Part model, mm, in its own coordinate system. A direction names the side the tool comes from. Give positions to 0.01 mm unless a question says otherwise; leave off trailing zeros. Write each loop counter-clockwise with the first axis right and the second up, starting at its lowest first coordinate (ties: lowest second). Pieces come first, ordered by that corner, then holes.
Autodesk Inventor part; units mm, degrees
ref_plane "YZ Plane" through (0, 0, 0) normal (1, 0, 0) x (0, 1, 0)
ref_plane "XZ Plane" through (0, 0, 0) normal (0, 1, 0) x (-1, 0, 0)
ref_plane "XY Plane" through (0, 0, 0) normal (0, 0, 1) x (1, 0, 0)
sketch "Esboço1" plane through (0, 0, 0) normal (0, 0, 1) x (1, 0, 0)
  circle A0 centre (0, 0) radius 10
  dimension "d0" = 20
extrude "Extrusão1" add sketch "Esboço1" along normal mid plane 300
sketch "Esboço2" plane through (0, 0, 150) normal (0, 0, 1) x (1, 0, 0)
  circle A0 centre (0, 0) radius 8
  dimension "d3" = 16
extrude "Extrusão2" add sketch "Esboço2" along normal blind 40
fillet "Arredondamento1" radius 2 1 edges at (-8, 0, 190)
mirror "Espelhamento1" about plane through (0, 0, 0) normal (0, 0, 1) of "Extrusão2", "Arredondamento1"
properties part number "Haste da Morsa"
1) Drill centre lines: L1, parallel to Z at x = 1, y = 9; L2, parallel to Y at x = -0.75, z = 60; L3, parallel to X at y = -0.75, z = 167.5. Where is each one in solid material? Low to high.
Check result:
L1: z = -150 to 150
L2: y = -9.97 to 9.97
L3: x = -7.96 to 7.96
2) 3-axis set-ups, long thin cutter, end or side, ignore diameter. For faces 1 (the cylindrical face through (-1.73, -7.81, -168.73)), 2 (the cylindrical face through (-1.73, 7.81, 168.73)), 3 (the cylindrical face through (-2.17, -9.76, 2.1)): which of +Z, -Z, +X, -X, +Y, -Y reach the whole face in a straight line?
Check result:
face 1: -Z
face 2: +Z
face 3: +Z, -Z
3) Saw through at A-A (x = 0). Write the cut outline in (y, z), and give its area (3 significant figures).
Check result:
outline: (-10, -150) - (-8, -150) - (-8, -188) arc R2 ccw to (-6, -190) - (6, -190) arc R2 ccw to (8, -188) - (8, -150) - (10, -150) - (10, 150) - (8, 150) - (8, 188) arc R2 ccw to (6, 190) - (-6, 190) arc R2 ccw to (-8, 188) - (-8, 150) - (-10, 150) - close
area: 7,280 mm2
4) Flat gauge pins, fed straight in: P1, Ø1.5, axis at y = -5, z = -121.5, coming from the +X side; P2, Ø12, axis at x = 6.5, z = -15.5, coming from the -Y side; P3, Ø10, axis at y = -7, z = -148.5, coming from the -X side. Where does each tip first touch, or does it go through?
Check result:
P1: stops at x = 9.05
P2: stops at y = -9.99
P3: stops at x = -9.8
5) Saw through at C-C (z = 55). Write the cut outline in (x, y).
Check result:
outline: circle Ø20 at (0, 0)
